For this review, use the dimensioned drawing (mm, ordinates from the lowest corner) and the shaded views. A direction names the side the tool comes from. Coordinates: 2 decimals unless noted, no trailing zeros. Loops run counter-clockwise (first coordinate to the right, second up) from the corner with the lowest first, then second, coordinate; pieces in that order, holes last. Notation, with made-up numbers: (71.5, 59.5) - (110.5, 59.5) arc R30 ccw to (110.5, 91.5) - close; hole circle Ø6 at (-38.5, 5.25). An arc over 180 degrees is marked (long way). Answer in a Markdown table with one row per item. Add a question column.
(1) For the marked faces 1 and 2, list the 3-axis set-ups (+Z, -Z, +X, -X, +Y, -Y) from which the entire face can be reached by the end or side of a thin tool; tool diameter is ignored.
(2) We need section C-C, the plane x = 1.25. Write out the cut boundary in (y, z).
(3) We need section A-A, the plane y = 2.5. Write out the cut boundary in (x, z), plus the area to 3 significant figures.
(4) To check wall thickness, follow L1, parallel to X at y = 2.9, z = 0.7; L2, parallel to Y at x = 4, z = 1.45; L3, parallel to Y at x = 2.75, z = 2.1 (1 decimal). State the ranges of each line that lie inside material, in increasing order. Write a range as [from, to].
(5) Clearance check with flat-ended pins moving along their axes: pin 1 (3 mm diameter, centred on x = 1.5, z = 1, fed in from -Y); pin 2 (1 mm diameter, centred on y = 4.5, z = 4, fed in from +X); pin 3 (2 mm diameter, centred on y = 3.5, z = 4.5, fed in from +X). State where each tip first meets the part, or that it passes through.
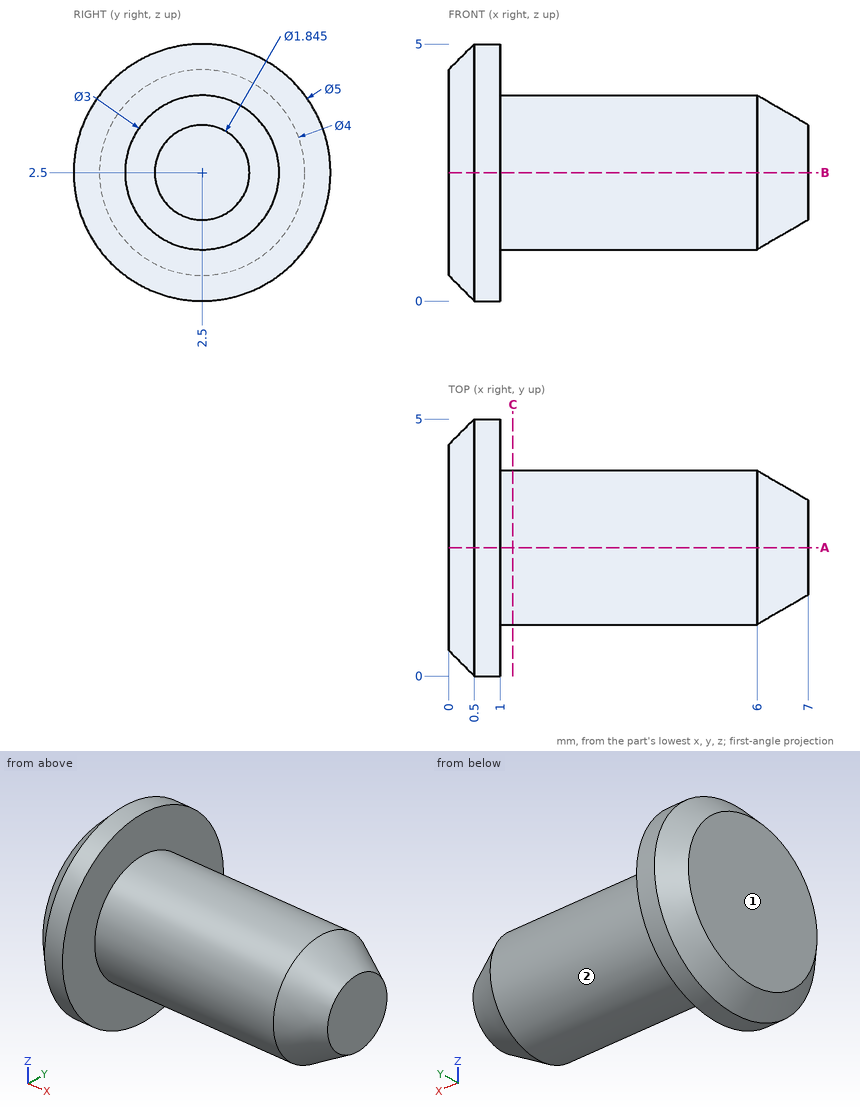
Responses:
| question | item | result |
|---|---|---|
| 1 | face 1 | +Z, -Z, -X, +Y, -Y |
| 1 | face 2 | +X |
| 2 | outline | circle Ø3 at (2.5, 2.5) |
| 3 | outline | (0, 0.5) - (0.5, 0) - (1, 0) - (1, 1) - (6, 1) - (7, 1.58) - (7, 3.42) - (6, 4) - (1, 4) - (1, 5) - (0.5, 5) - (0, 4.5) - close |
| 3 | area | 22.2 mm2 |
| 4 | L1 | x = [0, 1] |
| 4 | L2 | y = [1.43, 3.57] |
| 4 | L3 | y = [1.1, 3.9] |
| 5 | pin 1 | stops at y = 0 |
| 5 | pin 2 | stops at x = 1 |
| 5 | pin 3 | stops at x = 6.46 |
